from build123d import *

# Parameters (mm, degrees)
BOSS_EXTRUDE1_DEPTH            = 200
CUT_EXTRUDE1_START             = -6
CUT_EXTRUDE1_DEPTH             = 6
FILLET1_R                      = 1
FILLET2_R                      = 2.5
M5_CLEARANCE_HOLE1_D           = 5.5
M5_CLEARANCE_HOLE1_ON_FACE_2_D = 5.5


with BuildPart() as part:
    # Sketch1 → Boss-Extrude1 (new body)
    with BuildSketch(Plane(origin=(0, 0, 0), x_dir=(1, 0, 0), z_dir=(0, 1, 0))):
        with BuildLine():
            Line((0, 150), (0, 155))
            ThreePointArc((0, 155), (134.233937587, 77.5), (134.233937587, -77.5))
            Line((134.233937587, -77.5), (129.903810568, -75))
            ThreePointArc((129.903810568, -75), (129.903810568, 75), (0, 150))
        make_face()
    extrude(amount=BOSS_EXTRUDE1_DEPTH)

    # Sketch3 → Cut-Extrude1 (cut)
    with BuildSketch(Plane(origin=(0, 200, 0), x_dir=(1, 0, 0), z_dir=(0, 1, 0)).offset(CUT_EXTRUDE1_START)):
        with BuildLine():
            Line((21, 153.570830564), (21, 148.522725534))
            ThreePointArc((21, 148.522725534), (10.525948174, 149.630225606), (0, 150))
            Line((0, 150), (0, 155))
            ThreePointArc((0, 155), (10.524287687, 154.642294889), (21, 153.570830564))
        make_face()
        with BuildLine():
            Line((143.496240548, -58.598881802), (139.124453352, -56.074829287))
            ThreePointArc((139.124453352, -56.074829287), (134.846550636, -65.699374286), (129.903810568, -75))
            Line((129.903810568, -75), (134.233937587, -77.5))
            ThreePointArc((134.233937587, -77.5), (139.186299717, -68.206846951), (143.496240548, -58.598881802))
        make_face()
    extrude(amount=CUT_EXTRUDE1_DEPTH, mode=Mode.SUBTRACT)

    # Fillet1
    fillet1_edges = [part.edges().sort_by_distance(p)[0] for p in [
        (21, 194, -151.046778049),
        (141.31034695, 194, 57.336855545),
    ]]
    fillet(fillet1_edges, radius=FILLET1_R)

    # Fillet2
    fillet2_edges = [part.edges().sort_by_distance(p)[0] for p in [
        (134.233937587, 0, -77.5),
        (129.903810568, 0, -75),
    ]]
    fillet(fillet2_edges, radius=FILLET2_R - 0.0001)  # a hair under: the kernel refuses the full size

    # M5 Clearance Hole1 (through all)
    with Locations(Plane(origin=(138.954283246, 100, 68.678287453), x_dir=(-0.443085725506, 0, 0.89647924675), z_dir=(0.89647924675, 0, 0.443085725506))):
        with Locations((0, 0)):
            Hole(M5_CLEARANCE_HOLE1_D / 2)

    # M5 Clearance Hole1 on face 2 (through all)
    with Locations(Plane(origin=(10, 100, -154.677082983), x_dir=(-0.997916674108, 0, -0.064515978931), z_dir=(0.064515978931, 0, -0.997916674108))):
        with Locations((0, 0)):
            Hole(M5_CLEARANCE_HOLE1_ON_FACE_2_D / 2)


solid = part.part
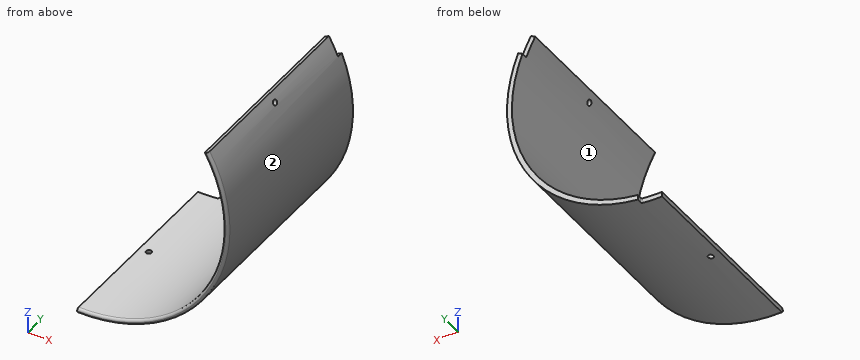
Read the model definition and answer for the solid it produces. Units are mm, in the model's axes. Face numbers are marked on the shaded views. Coordinates: 2 decimals unless noted, no trailing zeros. Loops run counter-clockwise (first coordinate to the right, second up) from the corner with the lowest first, then second, coordinate; pieces in that order, holes last.
Q1. The mould has two halves that part along Z. Classify the marked faces 1 and 2: +Z half, -Z half, draft (parallel to the pull), parting line (faces both ways), or undercut.
Q2. Each of these flat-tipped pins is pushed along its axis until it touches: pin 1 Ø5 at (x, z) = (11, -152.5) entering from +Y; pin 2 Ø2.5 at (y, z) = (198, -152) entering from -X; pin 3 Ø6 at (y, z) = (150.5, 23.5) entering from +X. Where does it stop, or does it pass through?
Q3. The part is cut by section A-A on y = 82.5. Write down the section's boundary in (x, z), and give its area (3 significant figures).
Q4. Consider probe 1 along Z at (x, y) = (21, 109); probe 2 along X at (y, z) = (10, 3.5); probe 3 along X at (y, z) = (90, 7.5). Determine where each line is inside the solid, lowest interval first.
Results below:
1. face 1: undercut
1. face 2: parting line
2. pin 1: stops at y = 194
2. pin 2: stops at x = 21
2. pin 3: stops at x = 153.64
3. outline: (0, -155) arc R155 ccw to (134.23, 77.5) - (129.9, 75) arc R150 cw to (0, -150) - close
3. area: 1,600 mm2
4. probe 1: z = -153.57 to -148.52
4. probe 2: x = 149.96 to 154.96
4. probe 3: x = 149.81 to 154.82
